from build123d import *

# Parameters (mm, degrees)
SKETCH_1_R          = 1.5
EXTRUDE_8_165_DEPTH = 2


with BuildPart() as part:
    # Эскиз1 → Бобышка8-165 (new body)
    with BuildSketch(Plane.XY):
        with BuildLine():
            Line((-10.301660458, -38.737628793), (-9.427477508, -36.938794679))
            ThreePointArc((-9.427477508, -36.938794679), (-10.221334445, -32.099598439), (-15.047492413, -31.229984527))
            ThreePointArc((-15.047492413, -31.229984527), (-18.460300533, -31.805984271), (-21.684930892, -30.54868796))
            ThreePointArc((-21.684930892, -30.54868796), (0, 34.75), (21.684930892, -30.54868796))
            ThreePointArc((21.684930892, -30.54868796), (18.460300533, -31.805984271), (15.047492413, -31.229984527))
            ThreePointArc((15.047492413, -31.229984527), (10.221334445, -32.099598439), (9.427477508, -36.938794679))
            Line((9.427477508, -36.938794679), (10.301660458, -38.737628793))
            ThreePointArc((10.301660458, -38.737628793), (11.313275299, -39.702001205), (12.709324487, -39.768524879))
            ThreePointArc((12.709324487, -39.768524879), (0, 41.75), (-12.709324487, -39.768524879))
            ThreePointArc((-12.709324487, -39.768524879), (-11.313275299, -39.702001205), (-10.301660458, -38.737628793))
        make_face()
        with Locations((-13.25, -35.08115591)):
            Circle(SKETCH_1_R, mode=Mode.SUBTRACT)
        with Locations(Location((13.25, -35.08115591, 0), (0, 0, 180))):
            Circle(SKETCH_1_R, mode=Mode.SUBTRACT)
    extrude(amount=EXTRUDE_8_165_DEPTH)


solid = part.part
Source: CAD feature listing. Evaluate the final solid. Frame: model axes, mm. A direction names the side the tool comes from. Coordinates: 2 decimals unless noted, no trailing zeros. Order: outer loops, then holes, each group sorted by start corner. A loop starts at its lowest first (then second) coordinate and runs counter-clockwise, first axis right, second up. Notation, with made-up numbers: M -22.75,44 L -0.75,44 A33 ccw -0.75,82 Z; hole C 47,40 d5. An arc over 180 degrees is marked long. Write each question's results on one line, items separated by ' | '. Start each with the question number.
Item 1: Line query: probe 1 along Y at (x, z) = (-13.5, 1.8); probe 2 along Y at (x, z) = (13.25, 1.55); probe 3 along X at (y, z) = (-4, 1.25). Output: solid intervals per line, ascending.
Item 2: Cut plane B-B (x = -29). Return loops of the section in (y, z), and give its area (3 significant figures).
Item 3: Cut plane D-D (x = 0). Return loops of the section in (y, z), and give its area (3 significant figures).
Item 4: Cut plane C-C (z = 0.4). Return loops of the section in (x, y).
Item 5: Draft query along Y for faces 4 (the face through (-18.41, -31.81, 0.99)), 5 (the face through (-11.33, -39.71, 0.99)), 6 (the face through (-6.4, 34.4, 0)), 7 (the face through (-1.269, 34.728, 0.986)). Return one class per face: pulls with the +Y half, pulls with the -Y half, needs draft (parallel to the pull), parting line crosses it, or undercut.
Item 6: Cut plane A-A (y = -15.5). Return loops of the section in (x, z).
Item 7: Set-up query: faces 1 (the face through (9.86, -37.83, 0.99)), 2 (the face through (18.5, -31.8, 1)), 3 (the face through (-6.4, 34.4, 2)). Return all of +Z, -Z, +X, -X, +Y, -Y with unobstructed straight access to the full face (end or side cutting, diameter ignored); none if empty.
Checked values:
1) probe 1: y = -39.51 to -36.56, -33.6 to -30.84, 32.14 to 39.51 | probe 2: y = -39.59 to -36.58, -33.58 to -30.83, 32.24 to 39.59 | probe 3: x = -41.56 to -36.16, 36.16 to 41.56
2) outline: M -30.03,0 L -23.25,0 L -23.25,2 L -30.03,2 Z; M 20.25,0 L 30.03,0 L 30.03,2 L 20.25,2 Z | area: 33.1 mm2
3) outline: M 34.75,0 L 41.75,0 L 41.75,2 L 34.75,2 Z | area: 14.0 mm2
4) outline: M -21.68,-30.55 A36.25 cw long 21.68,-30.55 A6.5 cw 15.05,-31.23 A4.25 ccw 9.43,-36.94 L 10.3,-38.74 A2 ccw 12.71,-39.77 A41.75 ccw long -12.71,-39.77 A2 ccw -10.3,-38.74 L -9.43,-36.94 A4.25 ccw -15.05,-31.23 A6.5 cw Z; hole C -13.25,-35.08 d3; hole C 13.25,-35.08 d3
5) face 4: undercut | face 5: pulls with the -Y half | face 6: needs draft | face 7: undercut
6) outline: M -38.77,0 L -33.44,0 L -33.44,2 L -38.77,2 Z; M 33.44,0 L 38.77,0 L 38.77,2 L 33.44,2 Z
7) face 1: +Z, -Z, -Y | face 2: +Z, -Z | face 3: +Z, +X, -X, +Y, -Y
